Here's the drawing with two shaded views (mm, measured from the low corner). I have some questions. Coordinates: 2 decimals unless noted, no trailing zeros. Loops run counter-clockwise (first coordinate to the right, second up) from the corner with the lowest first, then second, coordinate; pieces in that order, holes last. Notation, with made-up numbers: M 72.5,-16 L 123.5,-16 A16 cw 123.5,-1 Z; hole C -27.75,-20.5 d5. An arc over 180 degrees is marked long. Use one line per item in the form item = value. Start each with the question number.
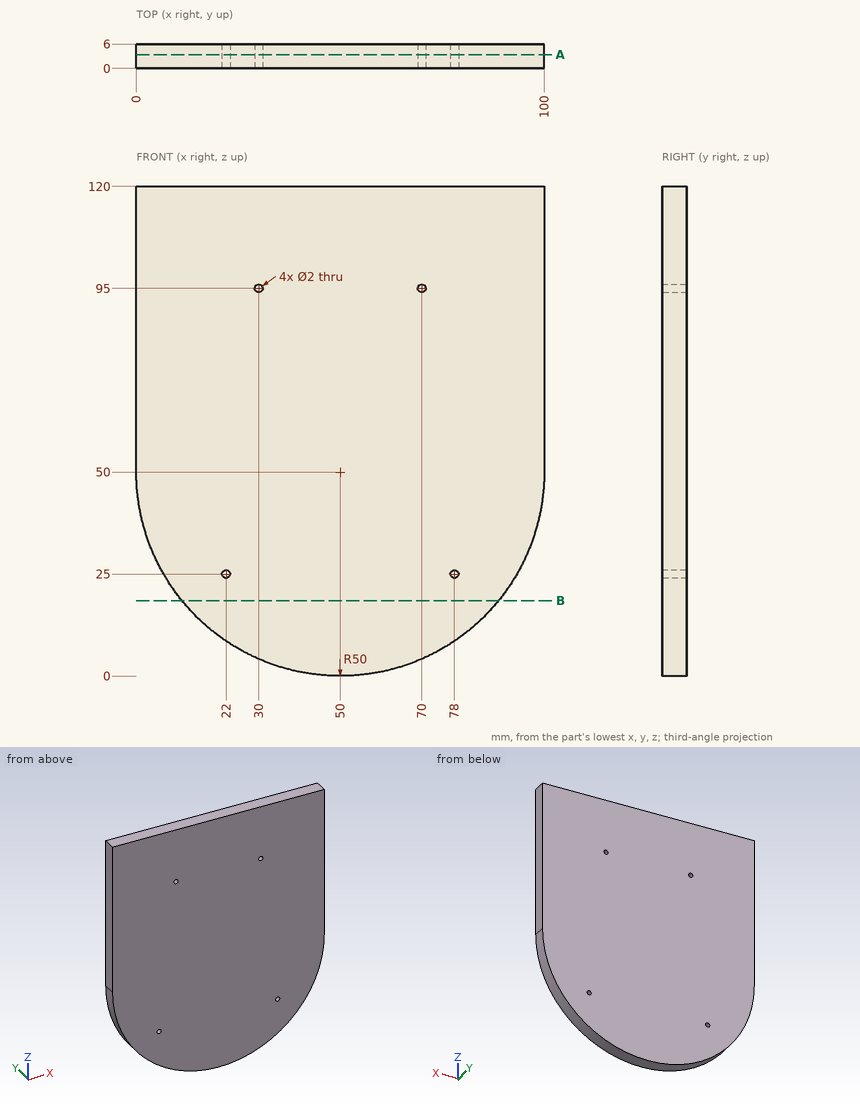
Item 1: I want a section at B-B (z = 18.5). Write out the boundary of the cut face in (x, y).
Item 2: I'm going to push flat-ended pins straight in: P1, Ø1.2, axis at x = 78, z = 25, coming from the +Y side; P2, Ø1.5, axis at y = 4, z = 27, coming from the +X side; P3, Ø3, axis at x = 77.5, y = 2.5, coming from the -Z side. Where does each tip first touch, or does it pass through?
Item 3: Please list where these lines run through material, in increasing order: line 1 along X through (y, z) = (2.6, 95); line 2 along X through (y, z) = (1.35, 25); line 3 along Z through (x, y) = (70, 4.2).
Item 4: I want a section at A-A (y = 3.4). Write out the boundary of the cut face in (x, z), plus the area to 3 significant figures.
Worked answers:
q1.outline = M 11.17,0 L 88.83,0 L 88.83,6 L 11.17,6 Z
q2.P1 = through
q2.P2 = 94.78
q2.P3 = 7.29
q3.line_1 = 0 to 29, 31 to 69, 71 to 100
q3.line_2 = 6.7 to 21, 23 to 77, 79 to 93.3
q3.line_3 = 4.17 to 94, 96 to 120
q4.outline = M 0,50 A50 ccw 100,50 L 100,120 L 0,120 Z; hole C 22,25 d2; hole C 30,95 d2; hole C 70,95 d2; hole C 78,25 d2
q4.area = 10,900 mm²
